Geometry check sheet. Reference: the model listing, model coordinates, mm. Give positions to 0.01 mm unless a question says otherwise; leave off trailing zeros. Write each loop counter-clockwise with the first axis right and the second up, starting at its lowest first coordinate (ties: lowest second). Pieces come first, ordered by that corner, then holes. Notation, with made-up numbers: (78.25, 9.5) - (126.25, 9.5) arc R16 cw to (126.25, 25.5) - close; hole circle Ø9 at (-20, 24.25). An arc over 180 degrees is marked (long way). Use a Markdown table: item, result.
```python
from build123d import *

# Parameters (mm, degrees)
SKETCH1_R                  = 7.5
BOSS_EXTRUDE1_DEPTH        = 10
CUT_EXTRUDE1_START         = -10
SKETCH2_R                  = 2.6
CUT_EXTRUDE1_DEPTH         = 10
CUT_EXTRUDE2_START         = -10
SKETCH3_R                  = 4.1
CUT_EXTRUDE2_DEPTH         = 10
F_2_7_2_7_DIAMETER_HOLE1_D = 2.7


with BuildPart() as part:
    # Sketch1 → Boss-Extrude1 (new, symmetric)
    with BuildSketch(Plane(origin=(0, 0, 0), x_dir=(1, 0, 0), z_dir=(0, 1, 0))):
        with Locations(Location((0, 0, 0), (0, 0, 270))):
            Circle(SKETCH1_R)
    extrude(amount=BOSS_EXTRUDE1_DEPTH, both=True)

    # Sketch2 → Cut-Extrude1 (cut)
    with BuildSketch(Plane(origin=(0, 10, 0), x_dir=(1, 0, 0), z_dir=(0, 1, 0)).offset(CUT_EXTRUDE1_START)):
        with Locations(Location((0, 0, 0), (0, 0, 270))):
            Circle(SKETCH2_R)
    extrude(amount=CUT_EXTRUDE1_DEPTH, mode=Mode.SUBTRACT)

    # Sketch3 → Cut-Extrude2 (cut)
    with BuildSketch(Plane.XZ.offset(10).offset(CUT_EXTRUDE2_START)):
        with Locations(Location((0, 0, 0), (0, 0, 270))):
            Circle(SKETCH3_R)
    extrude(amount=CUT_EXTRUDE2_DEPTH, mode=Mode.SUBTRACT)

    # Ø2.7 (2.7) Diameter Hole1 (through all)
    with Locations(Plane.XY.offset(10)):
        with Locations((0, 5), (0, -5)):
            Hole(F_2_7_2_7_DIAMETER_HOLE1_D / 2)


solid = part.part
```
1) Mould release check, pull along Z, two halves, no side actions. Record for faces 1 (the flat face through (-3, 0, 0)), 2 (the cylindrical face through (-1.57, -4.93, -3.787)), 3 (the flat face through (-3.2, -10, 3.2)), 4 (the cylindrical face through (-2.87, 0.14, 6.93)): pulls with the +Z half, pulls with the -Z half, needs draft (parallel to the pull), parting line crosses it, or undercut.
Working result:
| item | result |
|---|---|
| face 1 | undercut |
| face 2 | undercut |
| face 3 | needs draft |
| face 4 | parting line crosses it |
2) Section check B-B on z = 0. Record the boundary of the cut face in (x, y), then the cut area to 3 significant figures.
Working result:
| item | result |
|---|---|
| outline | (-7.5, -10) - (-4.1, -10) - (-4.1, 0) - (-2.6, 0) - (-2.6, 10) - (-7.5, 10) - close; (2.6, 0) - (4.1, 0) - (4.1, -10) - (7.5, -10) - (7.5, 10) - (2.6, 10) - close |
| area | 166 mm² |
3) Depth check by flat-ended pin: P1, Ø3, axis at x = -6, y = 1.5, coming from the -Z side; P2, Ø5, axis at y = 4.5, z = -4.5, coming from the -X side; P3, Ø6.5, axis at x = -0.5, z = 0.5, coming from the -Y side. Enter the tip coordinate at first touch or a pass-through.
Working result:
| item | result |
|---|---|
| P1 | stops at z = -6 |
| P2 | stops at x = -7.23 |
| P3 | stops at y = 0 |
4) Material ranges on L1, parallel to Y at x = 0, z = 4.4; L2, parallel to Y at x = 0, z = 3.65; L3, parallel to Z at x = 0.5, y = -1.5, recorded low to high. Write a range as from..to.
Working result:
| item | result |
|---|---|
| L1 | y = -10..-6.35, -3.65..3.65, 6.35..10 |
| L2 | y = 0..3.65, 6.35..10 |
| L3 | z = -7.48..-4.07, 4.07..7.48 |
5) Section check A-A on x = 0. Record the boundary of the cut face in (y, z), then the cut area to 3 significant figures.
Working result:
| item | result |
|---|---|
| outline | (-10, -7.5) - (-6.35, -7.5) - (-6.35, -4.1) - (-10, -4.1) - close; (-10, 4.1) - (-6.35, 4.1) - (-6.35, 7.5) - (-10, 7.5) - close; (-3.65, -7.5) - (3.65, -7.5) - (3.65, -2.6) - (0, -2.6) - (0, -4.1) - (-3.65, -4.1) - close; (-3.65, 4.1) - (0, 4.1) - (0, 2.6) - (3.65, 2.6) - (3.65, 7.5) - (-3.65, 7.5) - close; (6.35, -7.5) - (10, -7.5) - (10, -2.6) - (6.35, -2.6) - close; (6.35, 2.6) - (10, 2.6) - (10, 7.5) - (6.35, 7.5) - close |
| area | 121 mm² |
6) Section check C-C on y = -5. Record the boundary of the cut face in (x, z).
Working result:
| item | result |
|---|---|
| outline | (-1.35, -7.38) - (-1.35, -3.87) arc R4.1 cw to (-1.35, 3.87) - (-1.35, 7.38) arc R7.5 ccw to start; (1.35, -7.38) arc R7.5 ccw to (1.35, 7.38) - (1.35, 3.87) arc R4.1 cw to (1.35, -3.87) - close |
7) Section check D-D on z = 3.5. Record the boundary of the cut face in (x, y), then the cut area to 3 significant figures.
Working result:
| item | result |
|---|---|
| outline | (-6.63, -10) - (-2.14, -10) - (-2.14, 0) - (2.14, 0) - (2.14, -10) - (6.63, -10) - (6.63, 10) - (-6.63, 10) - close; hole circle Ø2.7 at (0, 5) |
| area | 217 mm² |
